```python
from build123d import *

# Parameters (mm, degrees)
SKETCH1_R           = 5
BOSS_EXTRUDE1_DEPTH = 3
SKETCH3_R           = 2.5
BOSS_EXTRUDE2_DEPTH = 18.5


with BuildPart() as part:
    # Sketch1 → Boss-Extrude1 (new body)
    with BuildSketch(Plane(origin=(0, 0, 0), x_dir=(0, 0, -1), z_dir=(1, 0, 0))):
        Circle(SKETCH1_R)
    extrude(amount=BOSS_EXTRUDE1_DEPTH)

    # Sketch3 → Boss-Extrude2 (add)
    with BuildSketch(Plane(origin=(3, 0, 0), x_dir=(0, 0, -1), z_dir=(1, 0, 0))):
        Circle(SKETCH3_R)
    extrude(amount=BOSS_EXTRUDE2_DEPTH)

    # Sketch4 → Revolve1 (revolve)
    with BuildSketch(Plane.XY, mode=Mode.PRIVATE) as revolve1_sk:
        Polygon((21.5, 0), (24, 0), (21.5, 2.5), align=None)
    revolve(revolve1_sk.sketch.rotate(Axis((21.5, 0, 0), (1, 0, 0)), 90), axis=Axis((21.5, 0, 0), (1, 0, 0)))


solid = part.part
```
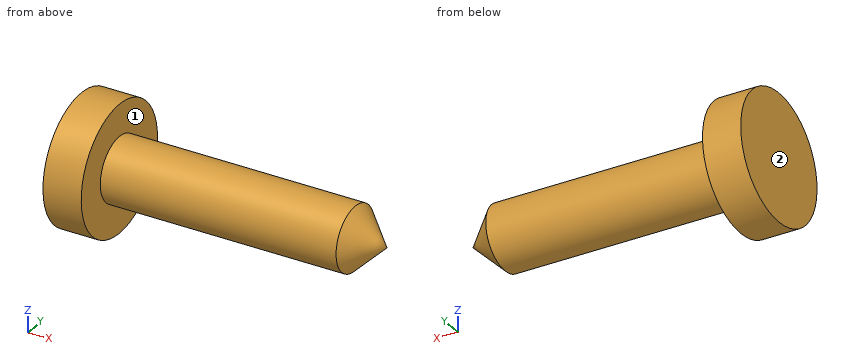
The listing builds one solid part. Answer for the finished solid, in the listing's coordinates (mm). Face numbers are marked on the shaded views. A direction names the side the tool comes from. Coordinates: 2 decimals unless noted, no trailing zeros. Loops run counter-clockwise (first coordinate to the right, second up) from the corner with the lowest first, then second, coordinate; pieces in that order, holes last. Notation, with made-up numbers: (77, -27.5) -> (93, -27.5) arc R21 ccw to (93, -20.5) -> close; hole circle Ø11 at (83.25, 57.25). An arc over 180 degrees is marked (long way). Return JSON: item names as keys, results as strings. Group by question number.
(1) Find the intervals of material crossed by probe 1 along X at (y, z) = (-1, -3.5); probe 2 along X at (y, z) = (-1.25, 0.5); probe 3 along Z at (x, y) = (3.75, -0.25), in increasing order. Write a range as from..to.
(2) Which of the six approach directions +Z, -Z, +X, -X, +Y, -Y give full straight-line access (tool end or side, diameter ignored) to the marked faces 1 and 2?
(3) A cutting plane is placed at B-B on x = 2.5. Write down the section's boundary in (y, z).
(4) Given pin 1 Ø4 at (y, z) = (-3, 1) entering from +X; pin 2 Ø3 at (x, y) = (14, -2) entering from +Z; pin 3 Ø1.5 at (x, y) = (6, 2) entering from -Z, each flat-ended and moving along its own axis, determine where each tip first touches the part or whether it passes through.
(5) A cutting plane is placed at C-C on y = 3.75. Write down the section's boundary in (x, z).
(6) A cutting plane is placed at A-A on z = 4. Write down the section's boundary in (x, y).
(7) A cutting plane is placed at D-D on x = 6.25. Write down the section's boundary in (y, z).
The answers:
{
 "1": {"probe 1": "x = 0..3", "probe 2": "x = 0..22.65", "probe 3": "z = -2.49..2.49"},
 "2": {"face 1": "+X", "face 2": "+Z, -Z, -X, +Y, -Y"},
 "3": {"outline": "circle Ø10 at (0, 0)"},
 "4": {"pin 1": "stops at x = 22.84", "pin 2": "stops at z = 2.45", "pin 3": "stops at z = -2.17"},
 "5": {"outline": "(0, -3.31) -> (3, -3.31) -> (3, 3.31) -> (0, 3.31) -> close"},
 "6": {"outline": "(0, -3) -> (3, -3) -> (3, 3) -> (0, 3) -> close"},
 "7": {"outline": "circle Ø5 at (0, 0)"}
}
